Could you check a few things on this model? Use its own coordinates, in mm. A direction names the side the tool comes from. Give positions to 0.01 mm unless a question says otherwise; leave off trailing zeros. Write each loop counter-clockwise with the first axis right and the second up, starting at its lowest first coordinate (ties: lowest second). Pieces come first, ordered by that corner, then holes. Notation, with made-up numbers: (79.5, -14.75) - (135.5, -14.75) arc R13 cw to (135.5, -10.75) - close; hole circle Ø6 at (38, 20.5). An arc over 180 degrees is marked (long way). Write item = value, one per line.
from build123d import *

# Parameters (mm, degrees)
BOSS_EXTRUDE1_REACH = 12.263
SKETCH4_R           = 2.475
BOSS_EXTRUDE2_REACH = 14.274
SKETCH1_R           = 3.2
CUT_EXTRUDE1_START  = -4
SKETCH5_R           = 2.475
CUT_EXTRUDE1_DEPTH  = 4
CUT_EXTRUDE2_REACH  = 14.274
SKETCH6_R           = 1.875


with BuildPart() as part:
    # Loft4: read off the stored shape, not the designer's step
    # Loft4: loft between two sections, ruled curve by curve
    loft4_from = [
        Edge.make_bspline([(3.50290491, 2.3, -1.597547242), (0.307810426, 2.3, -8.603357062), (-6.697999394, 2.3, -5.408262578), (-3.50290491, 2.3, 1.597547242), (-0.307810426, 2.3, 8.603357062), (6.697999394, 2.3, 5.408262578), (3.50290491, 2.3, -1.597547242)], [0, 0, 0, 0, 0.5, 0.5, 0.5, 1, 1, 1, 1], 3, [1, 0.333333333, 0.333333333, 1, 0.333333333, 0.333333333, 1]),
    ]
    loft4_to = [
        Edge.make_bspline([(2.465425341, 9.5, -0.414340307), (1.636744726, 9.5, -5.345190988), (-3.294105955, 9.5, -4.516510374), (-2.465425341, 9.5, 0.414340307), (-1.636744726, 9.5, 5.345190988), (3.294105955, 9.5, 4.516510374), (2.465425341, 9.5, -0.414340307)], [0, 0, 0, 0, 0.5, 0.5, 0.5, 1, 1, 1, 1], 3, [1, 0.333333333, 0.333333333, 1, 0.333333333, 0.333333333, 1]),
    ]
    loft4 = Solid(Shell([*[Face.make_surface_from_curves(loft4_from[k], loft4_to[k]) for k in range(1)], Face(Wire(loft4_from)), Face(Wire(loft4_to))]))
    add(loft4)

    # Sketch4 → Boss-Extrude1 (add, up to next)
    with BuildSketch(Plane(origin=(0, 11, 0), x_dir=(-1, 0, 0), z_dir=(0, 1, 0)), mode=Mode.PRIVATE) as boss_extrude1_sk1:
        with Locations(Location((0, 0, 0), (0, 0, 90))):
            Circle(SKETCH4_R)
    boss_extrude1_tool1 = extrude(boss_extrude1_sk1.sketch, amount=-BOSS_EXTRUDE1_REACH, mode=Mode.PRIVATE) - part.part
    add(boss_extrude1_tool1.solids().sort_by_distance((0, 11, 0))[0])

    # Sketch1 → Boss-Extrude2 (add, up to next)
    with BuildSketch(Plane(origin=(0, 0, 0), x_dir=(1, 0, 0), z_dir=(0, 1, 0)), mode=Mode.PRIVATE) as boss_extrude2_sk1:
        with Locations(Location((0, 0, 0), (0, 0, 90))):
            Circle(SKETCH1_R)
    boss_extrude2_tool1 = extrude(boss_extrude2_sk1.sketch, amount=BOSS_EXTRUDE2_REACH, mode=Mode.PRIVATE) - part.part
    add(boss_extrude2_tool1.solids().sort_by_distance((0, 0, 0))[0])

    # Sketch5 → Cut-Extrude1 (cut)
    with BuildSketch(Plane.XZ.offset(CUT_EXTRUDE1_START)):
        with Locations(Location((0, 0, 0), (0, 0, 90))):
            Circle(SKETCH5_R)
    extrude(amount=CUT_EXTRUDE1_DEPTH, mode=Mode.SUBTRACT)

    # Sketch6 → Cut-Extrude2 (cut, up to next)
    with BuildSketch(Plane(origin=(0, 11, 0), x_dir=(1, 0, 0), z_dir=(0, 1, 0)), mode=Mode.PRIVATE) as cut_extrude2_sk1:
        with Locations(Location((0, 0, 0), (0, 0, 270))):
            Circle(SKETCH6_R)
    cut_extrude2_tool1 = extrude(cut_extrude2_sk1.sketch, amount=-CUT_EXTRUDE2_REACH, mode=Mode.PRIVATE) & part.part
    add(cut_extrude2_tool1.solids().sort_by_distance((0, 11, 0))[0], mode=Mode.SUBTRACT)


solid = part.part
1. If we section it at B-B, the plane y = 10: Please give me the cut outline in (x, z) (3 decimals).
Filled sheet:
outline = circle Ø4.95 at (0, 0); hole circle Ø3.75 at (0, 0)
2. For pin 1 (1.5 mm diameter, centred on x = -1.5, y = 4, fed in from -Z); pin 2 (2 mm diameter, centred on x = 2.5, z = 0.5, fed in from -Y); pin 3 (1 mm diameter, centred on x = -2, y = 6, fed in from -Z); pin 4 (3 mm diameter, centred on x = 0, z = 0, fed in from +Y), each with a flat end and sliding along its axis, tell me the tip position at first contact or that it passes through.
Filled sheet:
pin_1 = -3.49
pin_2 = 0
pin_3 = -2.77
pin_4 = through
3. I need wall thicknesses on line 1 (X direction, y = 1.5, z = -2.25); line 2 (Z direction, x = 1, y = 9); line 3 (X direction, y = 1.9, z = 0) (3 decimals). Which ranges of each line are inside material? Lowest first, please.
Filled sheet:
line_1 = -2.28 to -1.03, 1.03 to 2.28
line_2 = -2.38 to -1.59, 1.59 to 2.38
line_3 = -3.2 to -2.475, 2.475 to 3.2
4. If we section it at A-A, the plane y = 2: Please give me the cut outline in (x, z) (3 decimals), and give its area (3 significant figures).
Filled sheet:
outline = circle Ø6.4 at (0, 0); hole circle Ø4.95 at (0, 0)
area = 12.9 mm2
5. Which directions (+Z, -Z, +X, -X, +Y, -Y) give clear straight access to the entire face, cutting with the end or side of a thin tool? Please do faces 1 (the face through (-2, 4, 1)), 2 (the face through (2, 11, 1)).
Filled sheet:
face_1 = -Y
face_2 = +Z, -Z, +X, -X, +Y
6. Thinking about a two-plate mould opening in Z: for faces 3 (the face through (0.74, 10.26, 2.36)), 4 (the face through (0.082, 7.549, -1.873)), 5 (the face through (2, 0, -2)), which applies, pulls with the +Z half, pulls with the -Z half, needs draft (parallel to the pull), parting line crosses it, or undercut?
Filled sheet:
face_3 = parting line crosses it
face_4 = undercut
face_5 = needs draft
